Read the model definition and answer for the solid it produces. Units are mm, in the model's axes. Face numbers are marked on the shaded views. A direction names the side the tool comes from. Coordinates: 2 decimals unless noted, no trailing zeros. Order: outer loops, then holes, each group sorted by start corner. A loop starts at its lowest first (then second) coordinate and runs counter-clockwise, first axis right, second up. Notation, with made-up numbers: (-20, -23.75) -> (23, -23.75) arc R31 ccw to (23, 3.25) -> close; hole circle Ø5 at (2, 0.5). An arc over 180 degrees is marked (long way). Answer in a Markdown table with one row per item.
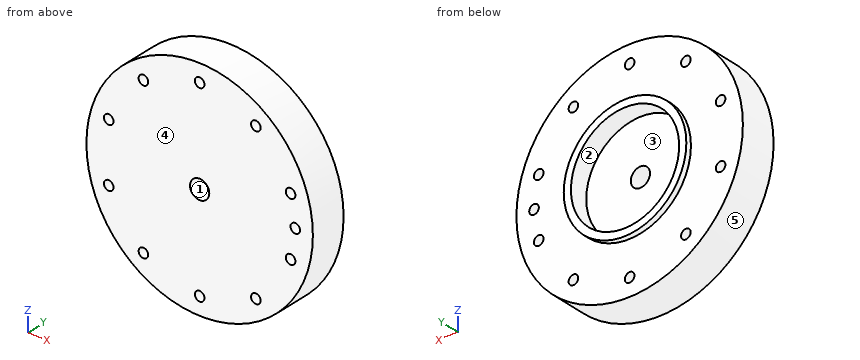
Autodesk Inventor part; units mm, degrees
ref_plane "YZ Plane" through (0, 0, 0) normal (1, 0, 0) x (0, 1, 0)
ref_plane "XZ Plane" through (0, 0, 0) normal (0, 1, 0) x (-1, 0, 0)
ref_plane "XY Plane" through (0, 0, 0) normal (0, 0, 1) x (1, 0, 0)
sketch "Sketch3" plane through (0, 0, 0) normal (0, 1, 0) x (-1, 0, 0)
  circle A0 centre (0, 0) radius 16.245
  circle A1 centre (0, -25.3377) radius 1.27
  circle A2 centre (-24.0976, -7.8298) radius 1.27
  circle A3 centre (-14.8931, 20.4986) radius 1.27
  circle A4 centre (24.0976, -7.8298) radius 1.27
  circle A5 centre (24.0976, 7.8298) radius 1.27
  circle A6 centre (-24.0976, 7.8298) radius 1.27
  circle A7 centre (-14.8931, -20.4986) radius 1.27
  circle A8 centre (0, 25.3377) radius 1.27
  circle A9 centre (14.8931, -20.4986) radius 1.27
  circle A10 centre (14.8931, 20.4986) radius 1.27
  circle A11 centre (-25.3377, 0) radius 1.27
  circle A12 centre (0, 0) radius 30
  circle A13 centre (0, 0) radius 16.245
  circle A14 centre (0, 0) radius 14.245
extrude "Extrusion4" add sketch "Sketch3" against normal blind 10 contours A0 | A12 | A14
extrude "Extrusion5" add sketch "Sketch3" along normal blind 1.5 contours A0
sketch "Sketch4" plane through (0, 1.5, 0) normal (0, 1, 0) x (1, 0, 0)
  circle A0 centre (0, 0) radius 14.245
  circle A1 centre (0, 0) radius 14.345
  dimension "d16" = 0.1
extrude "Extrusion7" cut sketch "Sketch4" against normal blind 5 contours A0 | A1
sketch "Sketch5" plane through (0, -3.5, 0) normal (0, 1, 0) x (1, 0, 0)
  circle A0 centre (0, 0) radius 2.55
  dimension "d19" = 5.1
extrude "Extrusion8" cut sketch "Sketch5" against normal up to surface (6.5 mm away)
properties part number "top"
Q1. The part is cut by section B-B (x = 0). Write down the section's boundary in (y, z) (3 decimals).
Outcome:
| item | result |
|---|---|
| outline | (-10, -30) -> (0, -30) -> (0, -26.608) -> (-10, -26.608) -> close; (-10, -24.068) -> (0, -24.068) -> (0, -16.245) -> (1.5, -16.245) -> (1.5, -14.345) -> (-3.5, -14.345) -> (-3.5, -2.55) -> (-10, -2.55) -> close; (-10, 2.55) -> (-3.5, 2.55) -> (-3.5, 14.345) -> (1.5, 14.345) -> (1.5, 16.245) -> (0, 16.245) -> (0, 24.068) -> (-10, 24.068) -> close; (-10, 26.608) -> (0, 26.608) -> (0, 30) -> (-10, 30) -> close |
Q2. For a pull along Z with two mould halves and no side action, classify the marked faces 3, 4 and 5 as pulls with the +Z half, pulls with the -Z half, needs draft (parallel to the pull), parting line crosses it, or undercut.
Outcome:
| item | result |
|---|---|
| face 3 | undercut |
| face 4 | needs draft |
| face 5 | parting line crosses it |
Q3. The part is cut by section A-A (z = 0). Write down the section's boundary in (x, y) (3 decimals), then the cut area to 3 significant figures.
Outcome:
| item | result |
|---|---|
| outline | (-30, -10) -> (-2.55, -10) -> (-2.55, -3.5) -> (-14.345, -3.5) -> (-14.345, 1.5) -> (-16.245, 1.5) -> (-16.245, 0) -> (-30, 0) -> close; (2.55, -10) -> (24.068, -10) -> (24.068, 0) -> (16.245, 0) -> (16.245, 1.5) -> (14.345, 1.5) -> (14.345, -3.5) -> (2.55, -3.5) -> close; (26.608, -10) -> (30, -10) -> (30, 0) -> (26.608, 0) -> close |
| area | 447 mm² |
Q4. Consider line 1 (Z direction, x = 0, y = -4.5); line 2 (Z direction, x = 0, y = 0.4) (3 decimals); line 3 (Z direction, x = 24.5, y = -5.75). Determine where each line is inside the solid, lowest interval first.
Outcome:
| item | result |
|---|---|
| line 1 | -30 to -26.61, -24.07 to -2.55, 2.55 to 24.07, 26.61 to 30 |
| line 2 | -16.245 to -14.345, 14.345 to 16.245 |
| line 3 | -17.31 to -9.03, -6.63 to -0.95, 0.95 to 6.63, 9.03 to 17.31 |
Q5. The part is cut by section D-D (x = -11). Write down the section's boundary in (y, z).
Outcome:
| item | result |
|---|---|
| outline | (-10, -27.91) -> (0, -27.91) -> (0, -11.95) -> (1.5, -11.95) -> (1.5, -9.21) -> (-3.5, -9.21) -> (-3.5, 9.21) -> (1.5, 9.21) -> (1.5, 11.95) -> (0, 11.95) -> (0, 27.91) -> (-10, 27.91) -> close |
Q6. For the marked faces 1 and 2, determine the directions among +Z, -Z, +X, -X, +Y, -Y from which every point of the face is accessible in a straight line to the end or side of a thin tool.
Outcome:
| item | result |
|---|---|
| face 1 | +Y, -Y |
| face 2 | +Y |
Q7. The part is cut by section C-C (y = -6.75). Give the number of separate pieces and of enclosed holes in the cut face, then the cut area to 3 significant figures.
Outcome:
| item | result |
|---|---|
| separate pieces | 1 |
| enclosed holes | 12 |
| area | 2,750 mm² |
Q8. Given pin 1 (4 mm diameter, centred on x = -21.5, z = 6, fed in from +Y); pin 2 (3 mm diameter, centred on x = -14.5, y = -2, fed in from -Z); pin 3 (2 mm diameter, centred on y = -3, z = -9.5, fed in from +X), each flat-ended and moving along its own axis, determine where each tip first touches the part or whether it passes through.
Outcome:
| item | result |
|---|---|
| pin 1 | y = 0 |
| pin 2 | z = -27.04 |
| pin 3 | x = 28.77 |
